Verification items for the finished model (mm, model axes). A direction names the side the tool comes from. Give positions to 0.01 mm unless a question says otherwise; leave off trailing zeros. Order: outer loops, then holes, each group sorted by start corner. A loop starts at its lowest first (then second) coordinate and runs counter-clockwise, first axis right, second up. Notation, with made-up numbers: (-33, 8.5) - (-10, 8.5) arc R3 ccw to (-10, 13.5) - close; hole circle Ø7 at (53.25, -10.75). An arc over 180 degrees is marked (long way). Answer as a JSON object with one key per item and string values.
```python
from build123d import *

# Parameters (mm, degrees)
BOSS_EXTRUDE1_DEPTH = 23
SKETCH3_W           = 102
SKETCH3_H           = 120
BOSS_EXTRUDE2_DEPTH = 4
SKETCH4_W           = 122
SKETCH4_H           = 120
CUT_EXTRUDE1_DEPTH  = 4
M16_TAPPED_HOLE1_D  = 14


with BuildPart() as part:
    # Sketch1 → Boss-Extrude1 (new body)
    with BuildSketch(Plane(origin=(0, 0, 0), x_dir=(1, 0, 0), z_dir=(0, 1, 0))):
        with BuildLine():
            Line((-95, 60), (95, 60))
            ThreePointArc((95, 60), (109.142135624, 54.142135624), (115, 40))
            Line((115, 40), (115, -40))
            ThreePointArc((115, -40), (109.142135624, -54.142135624), (95, -60))
            Line((95, -60), (-95, -60))
            ThreePointArc((-95, -60), (-109.142135624, -54.142135624), (-115, -40))
            Line((-115, -40), (-115, 40))
            ThreePointArc((-115, 40), (-109.142135624, 54.142135624), (-95, 60))
        make_face()
    extrude(amount=BOSS_EXTRUDE1_DEPTH)

    # Sketch3 → Boss-Extrude2 (add)
    with BuildSketch(Plane(origin=(0, 23, 0), x_dir=(1, 0, 0), z_dir=(0, 1, 0))):
        Rectangle(SKETCH3_W, SKETCH3_H)
    extrude(amount=BOSS_EXTRUDE2_DEPTH)

    # Sketch4 → Cut-Extrude1 (cut)
    with BuildSketch(Plane.XZ):
        Rectangle(SKETCH4_W, SKETCH4_H)
    extrude(amount=-CUT_EXTRUDE1_DEPTH, mode=Mode.SUBTRACT)

    # M16 Tapped Hole1 (through all)
    with Locations(Plane(origin=(-95, 23, -40), x_dir=(0, 0, 1), z_dir=(0, 1, 0))):
        with Locations((0, 0), (80, 0), (0, 190), (80, 190)):
            Hole(M16_TAPPED_HOLE1_D / 2)


solid = part.part
```
(1) Gauge pin test, flat ends, axial feed: pin 1 Ø22.5 at (x, z) = (-95, -40) entering from +Y; pin 2 Ø1.2 at (y, z) = (25.5, 0.5) entering from -X; pin 3 Ø2 at (y, z) = (24.5, 4) entering from +X. Record the tip position at first contact, or that the pin passes through.
Computed values:
{"pin 1": "stops at y = 23", "pin 2": "stops at x = -51", "pin 3": "stops at x = 51"}
(2) Access from +Z, -Z, +X, -X, +Y, -Y to the whole of each face (thin tool, end or side, straight path). Record for faces 4 (the flat face through (1, 13, 60)), 5 (the flat face through (83, 23, -1)), 6 (the cylindrical face through (-88.06, 11.34, -39.09)), 7 (the flat face through (-83, 23, -1)), 8 (the flat face through (61, 2, -1)).
Computed values:
{"face 4": "+Z, +X, -X, +Y, -Y", "face 5": "+Z, -Z, +X, +Y", "face 6": "+Y, -Y", "face 7": "+Z, -Z, -X, +Y", "face 8": "+Z, -Z, -Y"}
(3) Release check for a two-part mould opening along X. For faces 1 (the cylindrical face through (109.297, 11.339, 53.986)), 2 (the flat face through (-1, 4, 1)), 3 (the flat face through (-115, 11, 1)) record: pulls with the +X half, pulls with the -X half, needs draft (parallel to the pull), parting line crosses it, or undercut.
Computed values:
{"face 1": "pulls with the +X half", "face 2": "undercut", "face 3": "pulls with the -X half"}
(4) Section check B-B (z = 11). Record the cut outline in (x, y), then the cut area to 3 significant figures.
Computed values:
{"outline": "(-115, 0) - (-61, 0) - (-61, 4) - (61, 4) - (61, 0) - (115, 0) - (115, 23) - (51, 23) - (51, 27) - (-51, 27) - (-51, 23) - (-115, 23) - close", "area": "5,210 mm²"}
(5) Material ranges on line 1 along X through (y, z) = (16.25, 40); line 2 along X through (y, z) = (2, -5); line 3 along X through (y, z) = (16.5, 45), recorded low to high. Write a range as [from, to].
Computed values:
{"line 1": "x = [-115, -102], [-88, 88], [102, 115]", "line 2": "x = [-115, -61], [61, 115]", "line 3": "x = [-114.36, -99.9], [-90.1, 90.1], [99.9, 114.36]"}
(6) Section check D-D (x = -25). Record the cut outline in (y, z).
Computed values:
{"outline": "(4, -60) - (27, -60) - (27, 60) - (4, 60) - close"}
(7) Section check A-A (y = 20.5). Record the cut outline in (x, z), then the cut area to 3 significant figures.
Computed values:
{"outline": "(-115, -40) arc R20 ccw to (-95, -60) - (95, -60) arc R20 ccw to (115, -40) - (115, 40) arc R20 ccw to (95, 60) - (-95, 60) arc R20 ccw to (-115, 40) - close; hole circle Ø14 at (-95, -40); hole circle Ø14 at (-95, 40); hole circle Ø14 at (95, -40); hole circle Ø14 at (95, 40)", "area": "26,600 mm²"}
(8) Section check C-C (z = 44). Record the cut outline in (x, y).
Computed values:
{"outline": "(-114.6, 0) - (-100.74, 0) - (-100.74, 23) - (-114.6, 23) - close; (-89.26, 0) - (-61, 0) - (-61, 4) - (61, 4) - (61, 0) - (89.26, 0) - (89.26, 23) - (51, 23) - (51, 27) - (-51, 27) - (-51, 23) - (-89.26, 23) - close; (100.74, 0) - (114.6, 0) - (114.6, 23) - (100.74, 23) - close"}
